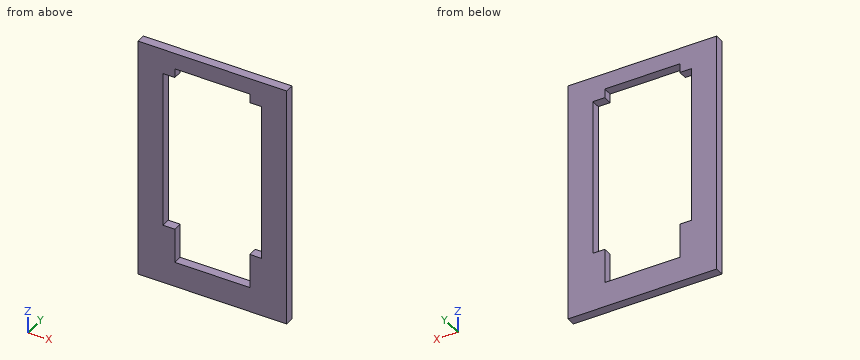
from build123d import *

# Parameters (mm, degrees)
SKETCH1_W           = 75.565
SKETCH1_H           = 105.41
SKETCH1_W_2         = 50.165
SKETCH1_H_2         = 80.01
BOSS_EXTRUDE1_DEPTH = 4.572
SKETCH2_W           = 38.1
SKETCH2_H           = 4.572
SKETCH2_H_2         = 8.128
CUT_EXTRUDE1_DEPTH  = 5.572
SKETCH3_W           = 38.1
SKETCH3_H           = 4.572
CUT_EXTRUDE2_DEPTH  = 5.572
SKETCH4_W           = 18.7325
SKETCH4_H           = 4.7625
BOSS_EXTRUDE2_DEPTH = 4.572


with BuildPart() as part:
    # Sketch1 → Boss-Extrude1 (new body)
    with BuildSketch(Plane(origin=(0, 0, 0), x_dir=(1, 0, 0), z_dir=(0, 1, 0))):
        Rectangle(SKETCH1_W, SKETCH1_H)
        Rectangle(SKETCH1_W_2, SKETCH1_H_2, mode=Mode.SUBTRACT)
    extrude(amount=BOSS_EXTRUDE1_DEPTH)

    # Sketch2 → Cut-Extrude1 (cut, through all)
    with BuildSketch(Plane(origin=(0, 4.572, 0), x_dir=(1, 0, 0), z_dir=(0, 1, 0))):
        with Locations((0, -42.291)):
            Rectangle(SKETCH2_W, SKETCH2_H)
        with Locations((0, 44.069)):
            Rectangle(SKETCH2_W, SKETCH2_H_2)
    extrude(amount=-CUT_EXTRUDE1_DEPTH, mode=Mode.SUBTRACT)

    # Sketch3 → Cut-Extrude2 (cut, through all)
    with BuildSketch(Plane(origin=(0, 4.572, 0), x_dir=(1, 0, 0), z_dir=(0, 1, 0))):
        with Locations((0, 50.419)):
            Rectangle(SKETCH3_W, SKETCH3_H)
    extrude(amount=-CUT_EXTRUDE2_DEPTH, mode=Mode.SUBTRACT)

    # Sketch4 → Boss-Extrude2 (add)
    with BuildSketch(Plane(origin=(0, 4.572, 0), x_dir=(1, 0, 0), z_dir=(0, 1, 0))):
        Polygon((-37.7825, 57.4675), (-19.05, 57.4675), (19.05, 57.4675), (37.7825, 57.4675), (37.7825, 70.1675), (-37.7825, 70.1675), align=None)
        with Locations((-28.41625, 55.08625)):
            Rectangle(SKETCH4_W, SKETCH4_H)
        with Locations((28.41625, 55.08625)):
            Rectangle(SKETCH4_W, SKETCH4_H)
    extrude(amount=-BOSS_EXTRUDE2_DEPTH)


solid = part.part
Part model, mm, in its own coordinate system. Give positions to 0.01 mm unless a question says otherwise; leave off trailing zeros. Loops run counter-clockwise (first coordinate to the right, second up) from the corner with the lowest first, then second, coordinate; pieces in that order, holes last. Notation, with made-up numbers: (32, -8.75) -> (89, -8.75) arc R17 cw to (89, 3.25) -> close; hole circle Ø7 at (47, 31). An arc over 180 degrees is marked (long way). Write each question's results on one line, items separated by ' | '. Start each with the question number.
Q1. Wall check: L1, parallel to X at y = 3.4, z = 27; L2, parallel to Z at x = -21, y = 2.9 (1 decimal); L3, parallel to X at y = 1.5, z = -42.5. Give the ranges that are in metal, low to high.
Q2. Band-saw the part on C-C on z = -12. List the corners of the cut face in (x, y), plus the area to 3 significant figures.
Q3. Band-saw the part on A-A on x = -21. List the corners of the cut face in (y, z) (1 decimal), plus the area to 3 significant figures.
Results are:
1) L1: x = -37.78 to -25.08, 25.08 to 37.78 | L2: z = -70.2 to -40, 40 to 52.7 | L3: x = -37.78 to -19.05, 19.05 to 37.78
2) outline: (-37.78, 0) -> (-25.08, 0) -> (-25.08, 4.57) -> (-37.78, 4.57) -> close; (25.08, 0) -> (37.78, 0) -> (37.78, 4.57) -> (25.08, 4.57) -> close | area: 116 mm²
3) outline: (0, -70.2) -> (4.6, -70.2) -> (4.6, -40) -> (0, -40) -> close; (0, 40) -> (4.6, 40) -> (4.6, 52.7) -> (0, 52.7) -> close | area: 196 mm²
